Source: three-view drawing plus pictorial views. Frame: mm from the lowest corner of the part. Round coordinates to 2 decimals unless told otherwise and drop trailing zeros. Write each loop counter-clockwise with the first axis right and the second up, starting at its lowest first coordinate (ties: lowest second). Pieces come first, ordered by that corner, then holes.
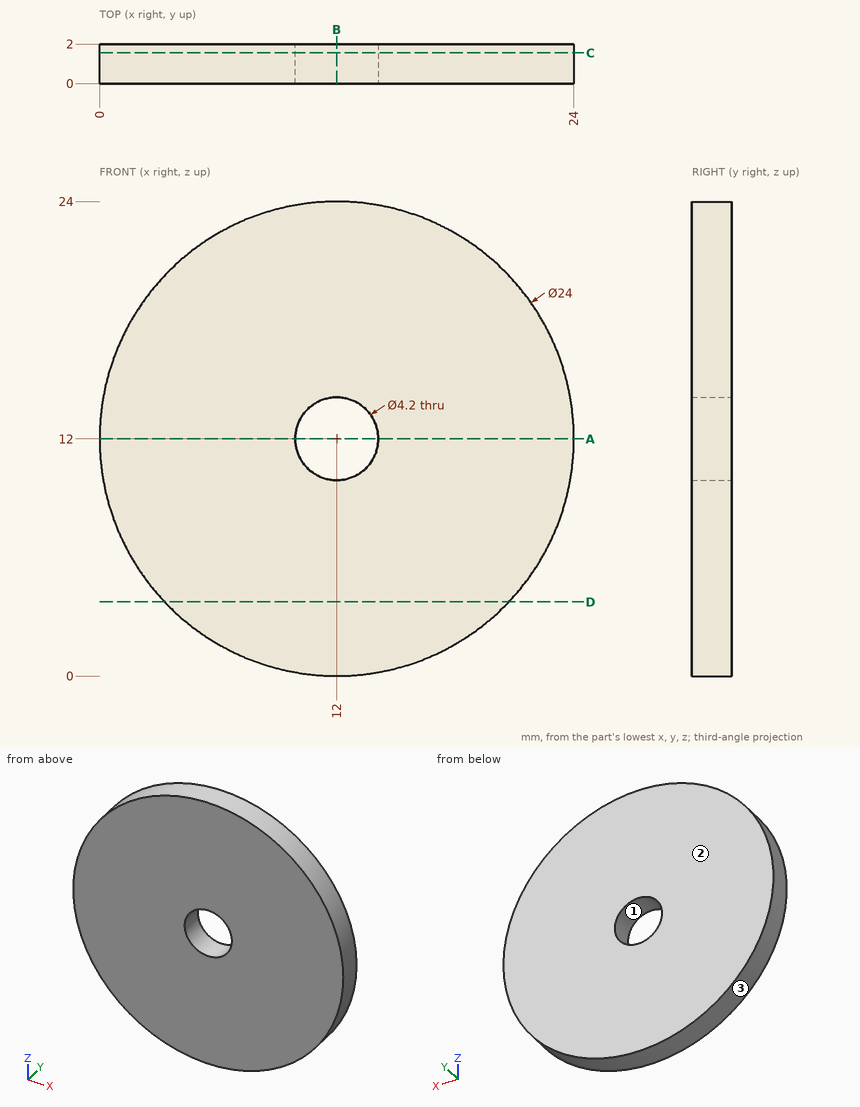
1) Section B-B on x = 12. Output: boundary loops of the cut face in (y, z).
2) Section C-C on y = 1.55. Output: boundary loops of the cut face in (x, z), plus the area to 3 significant figures.
3) Section D-D on z = 3.75. Output: boundary loops of the cut face in (x, y), plus the area to 3 significant figures.
4) Line query: probe 1 along Z at (x, y) = (12, 0.6); probe 2 along X at (y, z) = (1.1, 13); probe 3 along Z at (x, y) = (12.75, 1.6). Output: solid intervals per line, ascending.
5) Draft query along X for the marked faces 1, 2 and 3. Return one class per face: pulls with the +X half, pulls with the -X half, needs draft (parallel to the pull), parting line crosses it, or undercut.
6) Section A-A on z = 12. Output: boundary loops of the cut face in (x, y).
7) First-contact query: P1, Ø1, axis at x = 11, z = 13, coming from the -Y side. Flat tip, straight axial feed; report the tip coordinate or a pass-through.
Filled in:
1. outline: (0, 0) - (2, 0) - (2, 9.9) - (0, 9.9) - close; (0, 14.1) - (2, 14.1) - (2, 24) - (0, 24) - close
2. outline: circle Ø24 at (12, 12); hole circle Ø4.2 at (12, 12)
2. area: 439 mm2
3. outline: (3.29, 0) - (20.71, 0) - (20.71, 2) - (3.29, 2) - close
3. area: 34.9 mm2
4. probe 1: z = 0 to 9.9, 14.1 to 24
4. probe 2: x = 0.04 to 10.15, 13.85 to 23.96
4. probe 3: z = 0.02 to 10.04, 13.96 to 23.98
5. face 1: undercut
5. face 2: needs draft
5. face 3: parting line crosses it
6. outline: (0, 0) - (9.9, 0) - (9.9, 2) - (0, 2) - close; (14.1, 0) - (24, 0) - (24, 2) - (14.1, 2) - close
7. P1: passes through
